from build123d import *

# Parameters (mm, degrees)
SKETCH_1_W          = 232
SKETCH_1_H          = 40
SKETCH_1_R          = 2.1
EXTRUDE_2_DEPTH     = 5
SKETCH_3_R          = 2.1
CUT_EXTRUDE_2_DEPTH = 5
CUT_EXTRUDE_4_DEPTH = 5
FILLET_1_R          = 2


with BuildPart() as part:
    # 草图1 → 凸台-拉伸2 (new body)
    with BuildSketch(Plane.XY):
        Rectangle(SKETCH_1_W, SKETCH_1_H)
        with Locations((-46, 15)):
            Circle(SKETCH_1_R, mode=Mode.SUBTRACT)
        with Locations((46, 15)):
            Circle(SKETCH_1_R, mode=Mode.SUBTRACT)
        with Locations((46, -15)):
            Circle(SKETCH_1_R, mode=Mode.SUBTRACT)
        with Locations((-46, -15)):
            Circle(SKETCH_1_R, mode=Mode.SUBTRACT)
    extrude(amount=EXTRUDE_2_DEPTH)

    # 草图3 → 切除-拉伸2 (cut, symmetric)
    with BuildSketch(Plane.XY.offset(5)):
        with BuildLine():
            Line((-111, -15), (-111, 15))
            ThreePointArc((-111, 15), (-109.535533906, 18.535533906), (-106, 20))
            Line((-106, 20), (-116, 20))
            Line((-116, 20), (-116, -20))
            Line((-116, -20), (-106, -20))
            ThreePointArc((-106, -20), (-109.535533906, -18.535533906), (-111, -15))
        make_face()
        with Locations((-106, 15)):
            Circle(SKETCH_3_R)
        with Locations((-106, -15)):
            Circle(SKETCH_3_R)
        with BuildLine():
            Line((116, 20), (106, 20))
            ThreePointArc((106, 20), (109.535533906, 18.535533906), (111, 15))
            Line((111, 15), (111, -15))
            ThreePointArc((111, -15), (109.535533906, -18.535533906), (106, -20))
            Line((106, -20), (116, -20))
            Line((116, -20), (116, 20))
        make_face()
        with Locations((106, 15)):
            Circle(SKETCH_3_R)
        with Locations((106, -15)):
            Circle(SKETCH_3_R)
    extrude(amount=CUT_EXTRUDE_2_DEPTH, both=True, mode=Mode.SUBTRACT)

    # 草图4 → 切除-拉伸4 (cut, symmetric)
    with BuildSketch(Plane.XY.offset(5)):
        Polygon((-99.741377216, 14), (-76, 1.689656258), (-52.258622784, 14), align=None)
        Polygon((-103, 12.310343742), (-103, -12.310343742), (-79.258622784, 0), align=None)
        Polygon((-49, 12.310343742), (-72.741377216, 0), (-49, -12.310343742), align=None)
        Polygon((-76, -1.689656258), (-99.741377216, -14), (-52.258622784, -14), align=None)
        Polygon((-43, 12.422499667), (-43, -12.422499667), (-4.845179595, 0), align=None)
        Polygon((-38.154820405, 14), (0, 1.577500333), (38.154820405, 14), align=None)
        Polygon((43, 12.422499667), (4.845179595, 0), (43, -12.422499667), align=None)
        Polygon((0, -1.577500333), (-38.154820405, -14), (38.154820405, -14), align=None)
        Polygon((49, -12.310343742), (72.741377216, 0), (49, 12.310343742), align=None)
        Polygon((76, 1.689656258), (99.741377216, 14), (52.258622784, 14), align=None)
        Polygon((103, 12.310343742), (79.258622784, 0), (103, -12.310343742), align=None)
        Polygon((99.741377216, -14), (76, -1.689656258), (52.258622784, -14), align=None)
    extrude(amount=CUT_EXTRUDE_4_DEPTH, both=True, mode=Mode.SUBTRACT)

    # 圆角1
    fillet_1_edges = [part.edges().sort_by_distance(p)[0] for p in [
        (4.845179595, 0, 2.5),
        (43, 12.422499667, 2.5),
        (43, -12.422499667, 2.5),
        (0, 1.577500333, 2.5),
        (-38.154820405, 14, 2.5),
        (38.154820405, 14, 2.5),
        (-38.154820405, -14, 2.5),
        (0, -1.577500333, 2.5),
        (38.154820405, -14, 2.5),
        (49, -12.310343742, 2.5),
        (49, 12.310343742, 2.5),
        (72.741377216, 0, 2.5),
        (-103, -12.310343742, 2.5),
        (-103, 12.310343742, 2.5),
        (-79.258622784, 0, 2.5),
        (-72.741377216, 0, 2.5),
        (-49, 12.310343742, 2.5),
        (-49, -12.310343742, 2.5),
        (-76, -1.689656258, 2.5),
        (-52.258622784, -14, 2.5),
        (-99.741377216, -14, 2.5),
        (-43, -12.422499667, 2.5),
        (-43, 12.422499667, 2.5),
        (-4.845179595, 0, 2.5),
        (99.741377216, -14, 2.5),
        (52.258622784, -14, 2.5),
        (76, -1.689656258, 2.5),
        (99.741377216, 14, 2.5),
        (76, 1.689656258, 2.5),
        (52.258622784, 14, 2.5),
        (103, -12.310343742, 2.5),
        (79.258622784, 0, 2.5),
        (103, 12.310343742, 2.5),
        (-99.741377216, 14, 2.5),
        (-52.258622784, 14, 2.5),
        (-76, 1.689656258, 2.5),
    ]]
    fillet(fillet_1_edges, radius=FILLET_1_R)


solid = part.part
Verification items for the finished model (mm, model axes). A direction names the side the tool comes from. Round coordinates to 2 decimals unless told otherwise and drop trailing zeros. Order: outer loops, then holes, each group sorted by start corner. A loop starts at its lowest first (then second) coordinate and runs counter-clockwise, first axis right, second up.
1. Section check A-A on x = -46. Record the cut outline in (y, z).
Final values:
outline: (-20, 0) - (-17.1, 0) - (-17.1, 5) - (-20, 5) - close; (-12.9, 0) - (12.9, 0) - (12.9, 5) - (-12.9, 5) - close; (17.1, 0) - (20, 0) - (20, 5) - (17.1, 5) - close
2. Section check B-B on x = 67. Record the cut outline in (y, z), then the cut area to 3 significant figures.
Final values:
outline: (-20, 0) - (-14, 0) - (-14, 5) - (-20, 5) - close; (-6.36, 0) - (-2.98, 0) - (-2.98, 5) - (-6.36, 5) - close; (2.98, 0) - (6.36, 0) - (6.36, 5) - (2.98, 5) - close; (14, 0) - (20, 0) - (20, 5) - (14, 5) - close
area: 93.8 mm2
3. Section check D-D on x = -20. Record the cut outline in (y, z), then the cut area to 4 significant figures.
Final values:
outline: (-20, 0) - (-14, 0) - (-14, 5) - (-20, 5) - close; (-8.09, 0) - (-4.93, 0) - (-4.93, 5) - (-8.09, 5) - close; (4.93, 0) - (8.09, 0) - (8.09, 5) - (4.93, 5) - close; (14, 0) - (20, 0) - (20, 5) - (14, 5) - close
area: 91.55 mm2
4. Go/stop test with a flat-tipped pin: P1, Ø3, axis at x = -6.5, y = 6.5, coming from the -Z side. Record where the tip stops, or that it passes through.
Final values:
P1: passes through
5. Thickness scan on L1, parallel to X at y = -12, z = 4.3; L2, parallel to Y at x = -46, z = 2.45; L3, parallel to Y at x = 90, z = 0.7. Record the ranges inside material, lowest first.
Final values:
L1: x = -111 to -93.54, -58.46 to -27.55, 27.55 to 58.46, 93.54 to 111
L2: y = -20 to -17.1, -12.9 to 12.9, 17.1 to 20
L3: y = -20 to -14, -8.95 to -5.57, 5.57 to 8.95, 14 to 20
6. Access from +Z, -Z, +X, -X, +Y, -Y to the whole of each face (thin tool, end or side, straight path). Record for faces 1 (the cylindrical face through (-9.306, -0.035, 2.465)), 2 (the cylindrical face through (-110, 18, 2)).
Final values:
face 1: +Z, -Z
face 2: +Z, -Z, -X, +Y
7. Release check for a two-part mould opening along X. For faces 3 (the flat face through (-76, -14, 2)), 4 (the cylindrical face through (-43.997, 15.631, 2.465)), 5 (the flat face through (-1, 20, 2)), 6 (the cylindrical face through (-109, -19, 2)) record: +X half, -X half, draft (parallel to the pull), parting line (faces both ways), or undercut.
Final values:
face 3: undercut
face 4: undercut
face 5: draft
face 6: -X half
8. Section check C-C on z = 3.05. State how many separate pieces and enclosed holes the cut face has, then the cut area to 3 significant figures.
Final values:
separate pieces: 1
enclosed holes: 20
area: 4,740 mm2
